The model under review builds one solid part; all positions refer to its coordinate system, in mm. A direction names the side the tool comes from. Coordinates: 2 decimals unless noted, no trailing zeros. Write each loop counter-clockwise with the first axis right and the second up, starting at its lowest first coordinate (ties: lowest second). Pieces come first, ordered by that corner, then holes. Notation, with made-up numbers: M 64.25,-10.75 L 86.25,-10.75 A29 cw 86.25,10.25 Z; hole C -11.75,66 d11. An arc over 180 degrees is marked long. Answer as a JSON object with one key per item and string values.
Autodesk Inventor part; units mm, degrees
ref_plane "YZ Plane" through (0, 0, 0) normal (1, 0, 0) x (0, 1, 0)
ref_plane "XZ Plane" through (0, 0, 0) normal (0, 1, 0) x (-1, 0, 0)
ref_plane "XY Plane" through (0, 0, 0) normal (0, 0, 1) x (1, 0, 0)
sketch "Sketch1" plane through (0, 0, 0) normal (0, 1, 0) x (-1, 0, 0)
  line L0 (0, 0) -> (100, 0)
  line L1 (100, 0) -> (100, -100)
  line L2 (100, -100) -> (0, -100)
  line L3 (0, -100) -> (0, 0)
  dimension "d0" = 100
  dimension "d1" = 100
extrude "Extrusion1" add sketch "Sketch1" along normal blind 3.18
sketch "Sketch2" plane through (0, 0, 0) normal (0, 1, 0) x (-1, 0, 0)
  line L0 (100, 0) -> (0, 0)
  line L1 (0, 0) -> (0, -100)
  line L2 (0, -100) -> (100, -100)
  line L3 (100, -100) -> (100, 0)
  line L4 (-3.18, 0) -> (103.18, 0)
  line L5 (103.18, 0) -> (103.18, 3.18)
  line L6 (103.18, 3.18) -> (-3.18, 3.18)
  line L7 (-3.18, 3.18) -> (-3.18, 0)
  line L8 (103.18, -100) -> (-3.18, -100)
  line L9 (-3.18, -100) -> (-3.18, -103.18)
  line L10 (-3.18, -103.18) -> (103.18, -103.18)
  line L11 (103.18, -103.18) -> (103.18, -100)
  line L12 (103.18, 0) -> (100, 0)
  line L13 (100, 0) -> (100, -100)
  line L14 (100, -100) -> (103.18, -100)
  line L15 (103.18, -100) -> (103.18, 0)
  dimension "d4" = 3.18
  dimension "d5" = 3.18
  dimension "d6" = 3.18
  dimension "d7" = 3.18
extrude "Extrusion2" add sketch "Sketch2" along normal blind 70 contours L4 L15 L8 L3 | L0 L4 L7 L6 L5 | L8 L11 L10 L9 L2
properties part number "Base_caja"
(1) Wall thickness on line 1 along Z through (x, y) = (-25, 7); line 2 along Y through (x, z) = (-28, -56); line 3 along X through (y, z) = (52, -43.5): over which ranges is each line inside the solid? List them lowest first. Write a range as from..to.
Results list:
{"line 1": "-103.18..-100, 0..3.18", "line 2": "0..3.18", "line 3": "-103.18..-100"}
(2) For faces 1 (the face through (-100, 36, -51)), 2 (the face through (-103.18, 35, -51)), 3 (the face through (0, 2, -51)), list the 3-axis set-ups (+Z, -Z, +X, -X, +Y, -Y) from which the entire face can be reached by the end or side of a thin tool; tool diameter is ignored.
Results list:
{"face 1": "+X, +Y", "face 2": "+Z, -Z, -X, +Y, -Y", "face 3": "+X, +Y, -Y"}
(3) Add section C-C on z = -27. Give the boundary of the cut face in (x, y), and give its area (3 significant figures).
Results list:
{"outline": "M -103.18,0 L 0,0 L 0,3.18 L -100,3.18 L -100,70 L -103.18,70 Z", "area": "541 mm²"}
(4) Draft analysis for pull direction Z (two halves, no side actions). For faces 4 (the face through (-49, 3.18, -49)), 5 (the face through (-49, 0, -49)), 6 (the face through (-49, 35, -100)), 7 (the face through (-51, 35, 3.18)), state which applies: released by +Z, released by -Z, zero draft, split by the parting line, or undercut.
Results list:
{"face 4": "undercut", "face 5": "zero draft", "face 6": "undercut", "face 7": "released by +Z"}
(5) Add section B-B on y = 11.5. Give the boundary of the cut face in (x, z).
Results list:
{"outline": "M -103.18,-103.18 L 3.18,-103.18 L 3.18,-100 L -100,-100 L -100,0 L 3.18,0 L 3.18,3.18 L -103.18,3.18 Z"}
(6) Add section A-A on x = -88.5. Give the boundary of the cut face in (y, z).
Results list:
{"outline": "M 0,-103.18 L 70,-103.18 L 70,-100 L 3.18,-100 L 3.18,0 L 70,0 L 70,3.18 L 0,3.18 Z"}
(7) For pin 1 Ø2 at (x, z) = (-14.5, -86.5) entering from +Y; pin 2 Ø1 at (y, z) = (7.5, -15) entering from +X; pin 3 Ø1.6 at (y, z) = (1, -45.5) entering from +X, all flat-tipped, find the tip position at first contact; note any pin that passes through.
Results list:
{"pin 1": "y = 3.18", "pin 2": "x = -100", "pin 3": "x = 0"}
